```python
from build123d import *

# Parameters (mm, degrees)
BOSS_EXTRUDE1_DEPTH              = 38.1
F_1_8_0_125_DIAMETER_HOLE1_D     = 3.175
F_1_8_0_125_DIAMETER_HOLE1_DEPTH = 5.08
F_1_8_0_125_DIAMETER_HOLE1_TIP   = 0.953866233
F_1_8_0_15_DIAMETER_HOLE1_D      = 3.81
F_1_8_0_15_DIAMETER_HOLE1_DEPTH  = 5.08
F_1_8_0_15_DIAMETER_HOLE1_TIP    = 1.144639479


with BuildPart() as part:
    # Sketch1 → Boss-Extrude1 (new body)
    with BuildSketch(Plane.XY):
        with BuildLine():
            Line((5.08, 0), (67.31, 0))
            Line((67.31, 0), (67.31, 5.08))
            Line((67.31, 5.08), (10.16, 5.08))
            ThreePointArc((10.16, 5.08), (6.567897552, 6.567897552), (5.08, 10.16))
            Line((5.08, 10.16), (5.08, 46.99))
            Line((5.08, 46.99), (0, 46.99))
            Line((0, 46.99), (0, 5.08))
            ThreePointArc((0, 5.08), (1.487897552, 1.487897552), (5.08, 0))
        make_face()
    extrude(amount=BOSS_EXTRUDE1_DEPTH)

    # 1/8 (0.125) Diameter Hole1
    with Locations(Plane(origin=(0, 5.08, 0), x_dir=(1, 0, 0), z_dir=(0, 1, 0))):
        with Locations((62.103, -31.75), (62.103, -6.35)):
            Hole(F_1_8_0_125_DIAMETER_HOLE1_D / 2, depth=F_1_8_0_125_DIAMETER_HOLE1_DEPTH)
            with Locations((0, 0, -(F_1_8_0_125_DIAMETER_HOLE1_DEPTH + F_1_8_0_125_DIAMETER_HOLE1_TIP / 2))):  # 118° drill point
                Cone(0, F_1_8_0_125_DIAMETER_HOLE1_D / 2, F_1_8_0_125_DIAMETER_HOLE1_TIP, mode=Mode.SUBTRACT)

    # 1/8 (0.15) Diameter Hole1
    with Locations(Plane(origin=(5.08, 0, 0), x_dir=(0, 0, -1), z_dir=(1, 0, 0))):
        with Locations((-31.75, 40.64), (-6.35, 40.64), (-6.35, 21.59), (-31.75, 21.59)):
            Hole(F_1_8_0_15_DIAMETER_HOLE1_D / 2, depth=F_1_8_0_15_DIAMETER_HOLE1_DEPTH)
            with Locations((0, 0, -(F_1_8_0_15_DIAMETER_HOLE1_DEPTH + F_1_8_0_15_DIAMETER_HOLE1_TIP / 2))):  # 118° drill point
                Cone(0, F_1_8_0_15_DIAMETER_HOLE1_D / 2, F_1_8_0_15_DIAMETER_HOLE1_TIP, mode=Mode.SUBTRACT)


solid = part.part
```
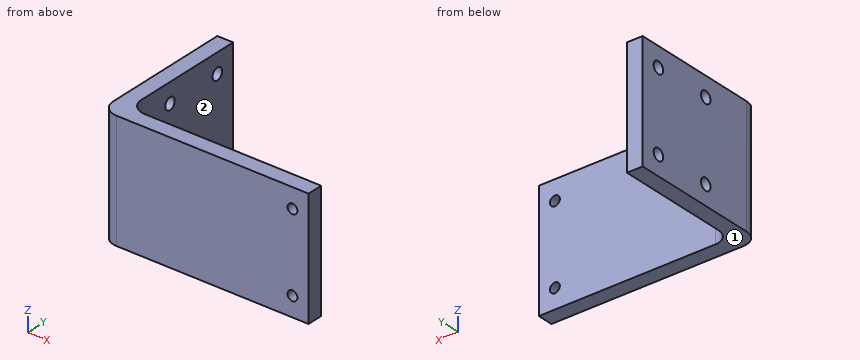
Input: part model. Units: mm. Frame: model coordinates. Face numbers are marked on the shaded views. A direction names the side the tool comes from. Coordinates: 2 decimals unless noted, no trailing zeros. Loops run counter-clockwise (first coordinate to the right, second up) from the corner with the lowest first, then second, coordinate; pieces in that order, holes last.
Q1. Section B-B, the plane y = 21.59. Return the cut outline in (x, z) (3 decimals), and give its area (3 significant figures).
Results are:
outline: (0, 0) - (5.08, 0) - (5.08, 4.445) - (0, 4.445) - close; (0, 8.255) - (5.08, 8.255) - (5.08, 29.845) - (0, 29.845) - close; (0, 33.655) - (5.08, 33.655) - (5.08, 38.1) - (0, 38.1) - close
area: 155 mm2
Q2. Section D-D, the plane x = 51. Return the cut outline in (y, z).
Results are:
outline: (0, 0) - (5.08, 0) - (5.08, 38.1) - (0, 38.1) - close
Q3. Section A-A, the plane z = 6.35. Return the cut outline in (x, y) (1 decimal).
Results are:
outline: (0, 5.1) arc R5.1 ccw to (5.1, 0) - (60.5, 0) - (60.5, 5.1) - (10.2, 5.1) arc R5.1 cw to (5.1, 10.2) - (5.1, 19.7) - (0, 19.7) - close; (0, 23.5) - (5.1, 23.5) - (5.1, 38.7) - (0, 38.7) - close; (0, 42.5) - (5.1, 42.5) - (5.1, 47) - (0, 47) - close; (63.7, 0) - (67.3, 0) - (67.3, 5.1) - (63.7, 5.1) - close
Q4. Line query: line 1 along Z through (x, y) = (1.1, 21.59) (3 decimals); line 2 along Y through (x, z) = (1.7, 31.75) (3 decimals); line 3 along Y through (x, z) = (3.35, 31.75) (3 decimals). Output: solid intervals per line, ascending.
Results are:
line 1: z = 0 to 4.445, 8.255 to 29.845, 33.655 to 38.1
line 2: y = 1.288 to 19.685, 23.495 to 38.735, 42.545 to 46.99
line 3: y = 0.304 to 19.685, 23.495 to 38.735, 42.545 to 46.99
Q5. Contact query for flat-ended pins moving along their axis: pin 1 (4.5 mm diameter, centred on y = 21.59, z = 6.35, fed in from -X); pin 2 (8 mm diameter, centred on x = 40.5, z = 29.5, fed in from +Y); pin 3 (12 mm diameter, centred on x = 15.5, y = 30.5, fed in from +Z); pin 4 (10 mm diameter, centred on y = 21, z = 26.5, fed in from +X). Output: stop coordinate, or through.
Results are:
pin 1: stops at x = 0
pin 2: stops at y = 5.08
pin 3: passes through
pin 4: stops at x = 5.08
Q6. Set-up query: the marked faces 1 and 2. Return all of +Z, -Z, +X, -X, +Y, -Y with unobstructed straight access to the full face (end or side cutting, diameter ignored); none if empty.
Results are:
face 1: -Z, +X, -X, +Y, -Y
face 2: +Z, -Z, +X, +Y
Q7. Section C-C, the plane z = 13. Return the cut outline in (x, y).
Results are:
outline: (0, 5.08) arc R5.08 ccw to (5.08, 0) - (67.31, 0) - (67.31, 5.08) - (10.16, 5.08) arc R5.08 cw to (5.08, 10.16) - (5.08, 46.99) - (0, 46.99) - close
